```python
from build123d import *

# Parameters (mm, degrees)
BOSS_EXTRUDE1_DEPTH  = 50
SKETCH2_R            = 2
CUT_EXTRUDE1_DEPTH   = 166.351141514
CUT_EXTRUDE2_DEPTH   = 10
BOSS_EXTRUDE3_DEPTH  = 5
MIRROR5_COPY_1_DEPTH = 5


with BuildPart() as part:
    # Sketch1 → Boss-Extrude1 (new body)
    with BuildSketch(Plane(origin=(0, 0, 0), x_dir=(1, 0, 0), z_dir=(0, 1, 0))):
        Polygon((0, 0), (125, 0), (125, 5), (5, 5), (5, 91), (125, 91), (125, 96), (0, 96), align=None)
    extrude(amount=BOSS_EXTRUDE1_DEPTH)

    # Sketch2 → Cut-Extrude1 (cut, through all)
    with BuildSketch(Plane.XY):
        with Locations((117, 25)):
            Circle(SKETCH2_R)
    extrude(amount=-CUT_EXTRUDE1_DEPTH, mode=Mode.SUBTRACT)

    # Sketch3 → Cut-Extrude2 (cut)
    with BuildSketch(Plane.XY):
        Polygon((52.5, 43.056819217), (33.609576666, 27.5), (52.5, 27.5), align=None)
        Polygon((50.140423334, 45), (12.359576666, 45), (31.25, 29.443180783), align=None)
        Polygon((28.890423334, 27.5), (10, 43.056819217), (10, 27.5), align=None)
        Polygon((10, 6.943180783), (28.890423334, 22.5), (10, 22.5), align=None)
        Polygon((12.359576666, 5), (50.140423334, 5), (31.25, 20.556819217), align=None)
        Polygon((52.5, 6.943180783), (52.5, 22.5), (33.609576666, 22.5), align=None)
        Polygon((57.5, 6.943180783), (76.390423334, 22.5), (57.5, 22.5), align=None)
        Polygon((59.859576666, 5), (97.640423334, 5), (78.75, 20.556819217), align=None)
        Polygon((81.109576666, 22.5), (100, 6.943180783), (100, 22.5), align=None)
        Polygon((100, 43.056819217), (81.109576666, 27.5), (100, 27.5), align=None)
        Polygon((97.640423334, 45), (59.859576666, 45), (78.75, 29.443180783), align=None)
        Polygon((76.390423334, 27.5), (57.5, 43.056819217), (57.5, 27.5), align=None)
        with BuildLine():
            Line((103.313708499, 50), (122.656854249, 30.656854249))
            ThreePointArc((122.656854249, 30.656854249), (124.39103626, 28.061467459), (125, 25))
            Line((125, 25), (125, 50))
            Line((125, 50), (103.313708499, 50))
        make_face()
        with BuildLine():
            Line((125, 0), (125, 25))
            ThreePointArc((125, 25), (124.39103626, 21.938532541), (122.656854249, 19.343145751))
            Line((122.656854249, 19.343145751), (103.313708499, 0))
            Line((103.313708499, 0), (125, 0))
        make_face()
    cut_extrude2 = extrude(amount=-CUT_EXTRUDE2_DEPTH, mode=Mode.SUBTRACT)

    # Mirror3: Cut-Extrude2 across plane
    add(cut_extrude2.mirror(Plane.XY.offset(-48)), mode=Mode.SUBTRACT)

    # Sketch6 → Boss-Extrude3 (add)
    with BuildSketch(Plane(origin=(0, 50, 0), x_dir=(1, 0, 0), z_dir=(0, 1, 0))):
        with BuildLine():
            Line((5, 5), (25, 5))
            ThreePointArc((25, 5), (10.857864376, 10.857864376), (5, 25))
            Line((5, 25), (5, 5))
        make_face()
    boss_extrude3 = extrude(amount=-BOSS_EXTRUDE3_DEPTH)

    # Mirror4: Boss-Extrude3 across plane
    add(boss_extrude3.mirror(Plane.ZX.offset(25)))

    # Mirror5: Boss-Extrude3 across plane
    add(boss_extrude3.mirror(Plane.XY.offset(-48)))

    # Mirror5 copy 1 sketch → Mirror5 copy 1 (add)
    with BuildSketch(Plane(origin=(0, 0, -96), x_dir=(1, 0, 0), z_dir=(0, -1, 0))):
        with BuildLine():
            Line((5, 5), (25, 5))
            ThreePointArc((25, 5), (10.857864376, 10.857864376), (5, 25))
            Line((5, 25), (5, 5))
        make_face()
    extrude(amount=-MIRROR5_COPY_1_DEPTH)


solid = part.part
```
Part model, mm, in its own coordinate system. A direction names the side the tool comes from. Round coordinates to 2 decimals unless told otherwise and drop trailing zeros. Loops run counter-clockwise (first coordinate to the right, second up) from the corner with the lowest first, then second, coordinate; pieces in that order, holes last.
Item 1: Drop flat-ended pins along their axis: P1, Ø1.5, axis at y = 33.5, z = -2, coming from the +X side; P2, Ø5.5, axis at y = 36.5, z = -93.5, coming from the +X side; P3, Ø1, axis at x = 13.5, y = 37, coming from the +Z side. Give the stop position or say it passes through.
Item 2: Cut at B-B, the plane x = 117. Give the cut face in (y, z).
Item 3: Cut at C-C, the plane z = -81. Give the cut face in (x, y), then the cut area to 3 significant figures.
Item 4: Mould opens along X. For faces 4 (the face through (113.121, 9.807, -2.465)), 5 (the face through (2, 50, -48)), 6 (the face through (10, 35, -94)) say: +X half, -X half, draft (parallel to the pull), parting line (faces both ways), or undercut.
Item 5: Cut at D-D, the plane y = 13. State how many separate pieces and enclosed holes the cut face has, then the cut area to 3 significant figures.
Item 6: Drill centre lines: line 1 (Z direction, x = 13, y = 44); line 2 (X direction, y = 16, z = -31); line 3 (Y direction, x = 117, z = -3.7). Where is each one in solid material? Low to high.
Item 7: Cut at A-A, the plane x = 8. Give the cut face in (y, z), then the cut area to 3 significant figures.
Item 8: 3-axis set-ups, long thin cutter, end or side, ignore diameter. For faces 1 (the face through (78, 5, -94)), 2 (the face through (113.121, 9.807, -93.535)), 3 (the face through (11.014, 47.535, -10.703)): which of +Z, -Z, +X, -X, +Y, -Y reach the whole face in a straight line?
A:
1. P1: stops at x = 120.56
1. P2: stops at x = 119.56
1. P3: passes through
2. outline: (13.69, -96) - (23, -96) - (23, -91) - (13.69, -91) - close; (13.69, -5) - (23, -5) - (23, 0) - (13.69, 0) - close; (27, -96) - (36.31, -96) - (36.31, -91) - (27, -91) - close; (27, -5) - (36.31, -5) - (36.31, 0) - (27, 0) - close
3. outline: (0, 0) - (7.68, 0) - (7.68, 5) - (5, 5) - (5, 45) - (7.68, 45) - (7.68, 50) - (0, 50) - close
3. area: 277 mm2
4. face 4: +X half
4. face 5: draft
4. face 6: undercut
5. separate pieces: 13
5. enclosed holes: 0
5. area: 932 mm2
6. line 1: z = -96 to -91, -5 to 0
6. line 2: x = 0 to 5
6. line 3: y = 13.69 to 23, 27 to 36.31
7. outline: (0, -96) - (50, -96) - (50, -81.54) - (45, -81.54) - (45, -91) - (5, -91) - (5, -81.54) - (0, -81.54) - close; (0, -14.46) - (5, -14.46) - (5, -5) - (45, -5) - (45, -14.46) - (50, -14.46) - (50, 0) - (0, 0) - close
7. area: 689 mm2
8. face 1: +Z, -Z
8. face 2: +Z, -Z, +X, -Y
8. face 3: +X, +Y, -Y
